Could you check a few things on this model? Use its own coordinates, in mm. A direction names the side the tool comes from. Give positions to 0.01 mm unless a question says otherwise; leave off trailing zeros. Loops run counter-clockwise (first coordinate to the right, second up) from the corner with the lowest first, then second, coordinate; pieces in that order, holes last.
1. Imagine slicing it at C-C (z = 9.25). List the corners of the cut face in (x, y) for me, plus the area to 3 significant figures.
2. For faces 1 (the flat face through (23, 0, -1)), 2 (the cylindrical face through (-13.22, -10.36, 23.49)), 3 (the flat face through (17, 7, 24.5)), which set-ups out of +Z, -Z, +X, -X, +Y, -Y let a thin tool reach every point of the face, with its end or its side?
3. Imagine slicing it at D-D (z = 20). List the corners of the cut face in (x, y) for me.
4. Imagine slicing it at A-A (y = 0). List the corners of the cut face in (x, z) for me.
5. For P1, Ø0.9, axis at x = 16, y = 9, coming from the +Z side; P2, Ø0.8, axis at y = 2.5, z = -1, coming from the -X side; P3, Ø2, axis at y = -7, z = 7.5, coming from the +X side; P4, Ø5, axis at x = 45.5, y = 5.5, coming from the +Z side, each with a flat end and sliding along its axis, tell me the tip position at first contact or that it passes through.
6. I need wall thicknesses on line 1 along Y through (x, z) = (-16.5, 23.65); line 2 along X through (y, z) = (8, 21); line 3 along Z through (x, y) = (45, -0.5). Which ranges of each line are inside material? Lowest first, please.
7. Imagine slicing it at B-B (x = -8). List the corners of the cut face in (y, z) for me.
8. Thinking about a two-plate mould opening in Y: for faces 4 (the flat face through (-16, -11, 24.5)), 5 (the cylindrical face through (58.45, 2.01, 2.86)), 6 (the flat face through (-17, -9, 22.5)), which applies, +Y half, -Y half, draft (parallel to the pull), parting line (faces both ways), or undercut?
```python
from build123d import *

# Parameters (mm, degrees)
SKETCH2_W           = 46
SKETCH2_H           = 32
BOSS_EXTRUDE1_DEPTH = 22.5
SKETCH3_R           = 3
BOSS_EXTRUDE2_DEPTH = 12
SKETCH4_R           = 3.55
SKETCH4_R_2         = 1.55
BOSS_EXTRUDE3_DEPTH = 2
SKETCH5_R           = 12
BOSS_EXTRUDE4_DEPTH = 32
SKETCH6_R           = 6.7
BOSS_EXTRUDE5_DEPTH = 7


with BuildPart() as part:
    # Sketch2 → Boss-Extrude1 (new body)
    with BuildSketch(Plane.XY):
        Rectangle(SKETCH2_W, SKETCH2_H)
    extrude(amount=BOSS_EXTRUDE1_DEPTH)

    # Sketch3 → Boss-Extrude2 (add)
    with BuildSketch(Plane.XY.offset(22.5)):
        with Locations((-8, 0)):
            Circle(SKETCH3_R)
    extrude(amount=BOSS_EXTRUDE2_DEPTH)

    # Sketch4 → Boss-Extrude3 (add)
    with BuildSketch(Plane.XY.offset(22.5)):
        with Locations((-16.5, 9)):
            Circle(SKETCH4_R)
        with Locations((-16.5, 9)):
            Circle(SKETCH4_R_2, mode=Mode.SUBTRACT)
        with Locations((-16.5, -9)):
            Circle(SKETCH4_R)
        with Locations((-16.5, -9)):
            Circle(SKETCH4_R_2, mode=Mode.SUBTRACT)
        with Locations((16.5, -9)):
            Circle(SKETCH4_R)
        with Locations((16.5, -9)):
            Circle(SKETCH4_R_2, mode=Mode.SUBTRACT)
        with Locations((16.5, 9)):
            Circle(SKETCH4_R)
        with Locations((16.5, 9)):
            Circle(SKETCH4_R_2, mode=Mode.SUBTRACT)
    extrude(amount=BOSS_EXTRUDE3_DEPTH)

    # Sketch5 → Boss-Extrude4 (add)
    with BuildSketch(Plane(origin=(23, 0, 0), x_dir=(0, 0, -1), z_dir=(1, 0, 0))):
        with Locations((-9.25, 0)):
            Circle(SKETCH5_R)
    extrude(amount=BOSS_EXTRUDE4_DEPTH)

    # Sketch6 → Boss-Extrude5 (add)
    with BuildSketch(Plane(origin=(55, 0, 0), x_dir=(0, 0, -1), z_dir=(1, 0, 0))):
        with Locations((-9.25, 0)):
            Circle(SKETCH6_R)
    extrude(amount=BOSS_EXTRUDE5_DEPTH)


solid = part.part
```
Derived:
1. outline: (-23, -16) - (23, -16) - (23, -12) - (55, -12) - (55, -6.7) - (62, -6.7) - (62, 6.7) - (55, 6.7) - (55, 12) - (23, 12) - (23, 16) - (-23, 16) - close
1. area: 2,330 mm2
2. face 1: -Z, -X, +Y, -Y
2. face 2: +Z
2. face 3: +Z, +X, -X, +Y, -Y
3. outline: (-23, -16) - (23, -16) - (23, -5.33) - (55, -5.33) - (55, 5.33) - (23, 5.33) - (23, 16) - (-23, 16) - close
4. outline: (-23, 0) - (23, 0) - (23, -2.75) - (55, -2.75) - (55, 2.55) - (62, 2.55) - (62, 15.95) - (55, 15.95) - (55, 21.25) - (23, 21.25) - (23, 22.5) - (-5, 22.5) - (-5, 34.5) - (-11, 34.5) - (-11, 22.5) - (-23, 22.5) - close
5. P1: stops at z = 22.5
5. P2: stops at x = 23
5. P3: stops at x = 62
5. P4: stops at z = 20.87
6. line 1: y = -12.55 to -10.55, -7.45 to -5.45, 5.45 to 7.45, 10.55 to 12.55
6. line 2: x = -23 to 23
6. line 3: z = -2.74 to 21.24
7. outline: (-16, 0) - (16, 0) - (16, 22.5) - (3, 22.5) - (3, 34.5) - (-3, 34.5) - (-3, 22.5) - (-16, 22.5) - close
8. face 4: draft
8. face 5: parting line
8. face 6: undercut
